Read the model definition and answer for the solid it produces. Units are mm, in the model's axes. A direction names the side the tool comes from. Round coordinates to 2 decimals unless told otherwise and drop trailing zeros. Loops run counter-clockwise (first coordinate to the right, second up) from the corner with the lowest first, then second, coordinate; pieces in that order, holes last. Notation, with made-up numbers: (-4, 59) - (11, 59) arc R9 cw to (11, 64) - close; hole circle Ø2 at (49, -20). An arc over 180 degrees is marked (long way). Use one line per item in the form item = value. Start each with the question number.
```python
from build123d import *

# Parameters (mm, degrees)
BOSS_EXTRUDE1_DEPTH = 16
SKETCH2_R           = 4.575
CUT_EXTRUDE1_DEPTH  = 2
CUT_EXTRUDE2_DEPTH  = 18.867638344
SKETCH5_W           = 9.1
SKETCH5_H           = 5
CUT_EXTRUDE4_DEPTH  = 18.867638344
SKETCH6_W           = 9.1
SKETCH6_H           = 2.5
CUT_EXTRUDE5_DEPTH  = 19.255204737


with BuildPart() as part:
    # Sketch1 → Boss-Extrude1 (new body)
    with BuildSketch(Plane.XY):
        Polygon((0, 0), (0, 0.95), (6, 0.95), (6, 0), (7.55, 0), (7.55, -0.8), (4.8, -3.55), (1.2, -3.55), (-1.55, -0.8), (-1.55, 0), align=None)
    extrude(amount=BOSS_EXTRUDE1_DEPTH)

    # Sketch2 → Cut-Extrude1 (cut)
    with BuildSketch(Plane(origin=(0, 0.95, 0), x_dir=(1, 0, 0), z_dir=(0, 1, 0))):
        with Locations((3, -8)):
            Circle(SKETCH2_R)
    extrude(amount=-CUT_EXTRUDE1_DEPTH, mode=Mode.SUBTRACT)

    # Sketch3 → Cut-Extrude2 (cut, through all)
    with BuildSketch(Plane(origin=(0, -1.05, 0), x_dir=(1, 0, 0), z_dir=(0, 1, 0))):
        Polygon((5.309401077, -8), (4.154700538, -6), (1.845299462, -6), (0.690598923, -8), (1.845299462, -10), (4.154700538, -10), align=None)
    extrude(amount=-CUT_EXTRUDE2_DEPTH, mode=Mode.SUBTRACT)

    # Sketch5 → Cut-Extrude4 (cut, through all)
    with BuildSketch(Plane(origin=(0, -1.05, 0), x_dir=(1, 0, 0), z_dir=(0, 1, 0))):
        with Locations((3, -8)):
            Rectangle(SKETCH5_W, SKETCH5_H)
    extrude(amount=CUT_EXTRUDE4_DEPTH, mode=Mode.SUBTRACT)

    # Sketch6 → Cut-Extrude5 (cut, through all)
    with BuildSketch(Plane(origin=(0, 0.95, 0), x_dir=(1, 0, 0), z_dir=(0, 1, 0))):
        with Locations((3, -1.25)):
            Rectangle(SKETCH6_W, SKETCH6_H)
        with Locations((3, -14.75)):
            Rectangle(SKETCH6_W, SKETCH6_H)
    extrude(amount=-CUT_EXTRUDE5_DEPTH, mode=Mode.SUBTRACT)


solid = part.part
```
1) For faces 4 (the flat face through (-0.16, -2.19, 7.92)), 5 (the flat face through (0, 0.5, 12.5)), 6 (the flat face through (4.724, -2.282, 9.014)), 7 (the flat face through (7, 0, 4)), 8 (the flat face through (3, -1, 13.5)), determine the directions among +Z, -Z, +X, -X, +Y, -Y from which every point of the face is accessible in a straight line to the end or side of a thin tool.
2) Determine the mould class of faces 1 (the flat face through (3, -1, 2.5)), 2 (the cylindrical face through (2.936, -0.036, 12.575)), 3 (the flat face through (3, -3.55, 12)) for opening direction Z: +Z half, -Z half, draft (parallel to the pull), parting line (faces both ways), or undercut.
3) A cutting plane is placed at C-C on z = 6.25. Write down the section's boundary in (x, y), plus the area to 3 significant figures.
4) A cutting plane is placed at B-B on y = -1.55. Write down the section's boundary in (x, z), plus the area to 3 significant figures.
5) A cutting plane is placed at A-A on x = 3. Write down the section's boundary in (y, z) (3 decimals), plus the area to 3 significant figures.
6) A cutting plane is placed at D-D on z = 12. Write down the section's boundary in (x, y).
7) Straight lines are drawn through the part: line 1 (Z direction, x = 3.5, y = -2.95); line 2 (X direction, y = -3.2, z = 6.25); line 3 (Y direction, x = 3.5, z = 4). For each, find the intervals that lie inside material, in ascending order. Write a range as from..to.
8) Flat-ended cylindrical pins translate along their axes: pin 1 (0.8 mm diameter, centred on y = 0.5, z = 4, fed in from +X); pin 2 (0.8 mm diameter, centred on x = 6.5, z = 3.5, fed in from +Y); pin 3 (0.5 mm diameter, centred on y = 0.5, z = 13, fed in from -X). Find the tip coordinate at first contact, or state that the pin passes through.
Checks:
q1.face_4 = +Z, -Z, -X, -Y
q1.face_5 = +Z, -Z, -X, +Y
q1.face_6 = +Y, -Y
q1.face_7 = +Z, -Z, +X, +Y
q1.face_8 = +Z, +X, -X, +Y, -Y
q2.face_1 = -Z half
q2.face_2 = undercut
q2.face_3 = draft
q3.outline = (-1.3, -1.05) - (1.2, -3.55) - (1.7, -3.55) - (1.7, -1.05) - close; (4.3, -3.55) - (4.8, -3.55) - (7.3, -1.05) - (4.3, -1.05) - close
q3.area = 8.75 mm²
q4.outline = (-0.8, 2.5) - (6.8, 2.5) - (6.8, 13.5) - (-0.8, 13.5) - close; hole (0.69, 8) - (1.85, 6) - (4.15, 6) - (5.31, 8) - (4.15, 10) - (1.85, 10) - close
q4.area = 69.7 mm²
q5.outline = (-3.55, 2.5) - (0.95, 2.5) - (0.95, 3.425) - (-1.05, 3.425) - (-1.05, 6) - (-3.55, 6) - close; (-3.55, 10) - (-1.05, 10) - (-1.05, 12.575) - (0.95, 12.575) - (0.95, 13.5) - (-3.55, 13.5) - close
q5.area = 21.2 mm²
q6.outline = (-1.55, -0.8) - (1.2, -3.55) - (4.8, -3.55) - (7.55, -0.8) - (7.55, 0) - (6, 0) - (6, 0.95) - (5.22, 0.95) - (5.22, -1.05) - (0.78, -1.05) - (0.78, 0.95) - (0, 0.95) - (0, 0) - (-1.55, 0) - close
q7.line_1 = 2.5..6, 10..13.5
q7.line_2 = 0.85..1.7, 4.3..5.15
q7.line_3 = -3.55..-1.05
q8.pin_1 = 6
q8.pin_2 = 0
q8.pin_3 = 0
